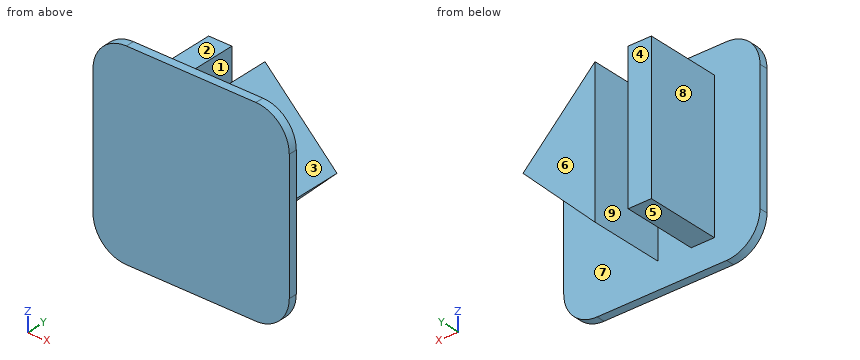
Autodesk Inventor part; units mm, degrees
ref_plane "YZ Plane" through (0, 0, 0) normal (1, 0, 0) x (0, 1, 0)
ref_plane "XZ Plane" through (0, 0, 0) normal (0, 1, 0) x (-1, 0, 0)
ref_plane "XY Plane" through (0, 0, 0) normal (0, 0, 1) x (1, 0, 0)
sketch "Szkic1" plane through (0, 0, 0) normal (0, 1, 0) x (-1, 0, 0)
  line L0 (5.1235, 4.3458) -> (-4.6765, 4.3458)
  line L1 (-4.6765, 4.3458) -> (-4.6765, -5.4542)
  line L2 (-4.6765, -5.4542) -> (5.1235, -5.4542)
  line L3 (5.1235, -5.4542) -> (5.1235, 4.3458)
  line L4 (5.1235, 4.3458) -> (-4.6765, -5.4542) construction
  line L5 (-4.6765, 4.3458) -> (5.1235, -5.4542) construction
  line L6 (0.2235, -0.5542) -> (2.6735, -0.5542)
  line L7 (3.4085, 3.8558) -> (1.9385, 3.8558)
  line L8 (1.9385, 3.8558) -> (1.9385, -4.9642)
  line L9 (1.9385, -4.9642) -> (3.4085, -4.9642)
  line L10 (3.4085, -4.9642) -> (3.4085, 3.8558)
  line L11 (3.4085, 3.8558) -> (1.9385, -4.9642) construction
  line L12 (1.9385, 3.8558) -> (3.4085, -4.9642) construction
  line L13 (0.2235, -0.5542) -> (0.0314, -0.5542)
  line L14 (0.0314, -0.5542) -> (0.0314, -4.9642)
  line L15 (0.0314, -0.5542) -> (-4.3786, -0.5542)
  line L16 (-4.3786, -0.5542) -> (0.0314, -4.9642)
  line L17 (-4.3786, -0.5542) -> (0.0314, 3.8558)
  line L18 (0.0314, -0.5542) -> (0.0314, 3.8558)
  line L19 (-5.6565, 5.3258) -> (6.1035, 5.3258)
  line L20 (6.1035, 5.3258) -> (6.1035, -6.4342)
  line L21 (6.1035, -6.4342) -> (-5.6565, -6.4342)
  line L22 (-5.6565, -6.4342) -> (-5.6565, 5.3258)
  line L23 (-5.6565, 5.3258) -> (6.1035, -6.4342) construction
  line L24 (6.1035, 5.3258) -> (-5.6565, -6.4342) construction
  point P0 (0, 0)
  dimension "d0" = 9.8
  dimension "d1" = 9.8
  dimension "d2" = 2.45
  dimension "d3" = 1.47
  dimension "d4" = 8.82
  dimension "d5" = 0.1921
  dimension "d6" = 4.41
  dimension "d7" = 4.41
  dimension "d8" = 11.76
  dimension "d9" = 11.76
extrude "Wyciągnięcie proste1" add sketch "Szkic1" along normal blind 0.5 contours L3 L2 L1 L0 | L10 L9 L8 L7 | L14 L16 L15 | L15 L17 L18 | L19 L20 L21 L22
extrude "Wyciągnięcie proste2" add sketch "Szkic1" along normal blind 5 contours L10 L9 L8 L7 | L14 L16 L15 | L15 L17 L18
fillet "Zaokrąglenie1" radius 2 4 edges at (5.6565, 0.25, 5.3258) (-6.1035, 0.25, 5.3258) (5.6565, 0.25, -6.4342) (-6.1035, 0.25, -6.4342)
offset faces "Rozmiar1" outward -0.04 faces at (-1.9385, 2, 0.9158) (-2.4285, 2, -4.9642) (-3.4085, 2, -2.0242) (-2.9185, 2, 3.8558) (-0.0314, 2, -2.0242) (1.4386, 2, 2.3858) (2.9086, 2, -2.0242)
properties part number "guzik_stop"
The model under review builds one solid part; all positions refer to its coordinate system, in mm. Face numbers are marked on the shaded views. A direction names the side the tool comes from. Coordinates: 2 decimals unless noted, no trailing zeros. Write each loop counter-clockwise with the first axis right and the second up, starting at its lowest first coordinate (ties: lowest second). Pieces come first, ordered by that corner, then holes. Notation, with made-up numbers: (25.5, -19) - (61.5, -19) arc R10 cw to (61.5, 0) - close; hole circle Ø6 at (17.5, 9). An arc over 180 degrees is marked (long way). Answer as CSV lines item,"result".
(1) We need section B-B (x = -2.5). Give the boundary of the cut face in (y, z).
Data:
outline,"(0, -6.43) - (0.5, -6.43) - (0.5, -4.92) - (5, -4.92) - (5, 3.82) - (0.5, 3.82) - (0.5, 5.33) - (0, 5.33) - close"
(2) Mouldability with a two-part tool opening along X and no side actions: class the marked faces 6, 7, 8 and 9 as pulls with the +X half, pulls with the -X half, needs draft (parallel to the pull), parting line crosses it, or undercut.
Data:
face 6,"needs draft"
face 7,"undercut"
face 8,"pulls with the -X half"
face 9,"undercut"
(3) We need section A-A (y = 2.85). Give the boundary of the cut face in (x, z), plus the area to 3 significant figures.
Data:
outline,"(-3.37, -4.92) - (-1.98, -4.92) - (-1.98, 3.82) - (-3.37, 3.82) - close; (0.01, -4.87) - (4.32, -0.55) - (0.01, 3.76) - close"
area,"30.8 mm2"
(4) We need section D-D (x = 2). Give the boundary of the cut face in (y, z), plus the area to 3 significant figures.
Data:
outline,"(0, -6.43) - (0.5, -6.43) - (0.5, -2.88) - (5, -2.88) - (5, 1.77) - (0.5, 1.77) - (0.5, 5.33) - (0, 5.33) - close"
area,"26.8 mm2"
(5) Tool access review of the marked faces 1, 2, 3, 4 and 5: name each direction out of +Z, -Z, +X, -X, +Y, -Y from which nothing blocks a thin tool from reaching the whole face with its end or side.
Data:
face 1,"+Z, -Z, +Y"
face 2,"+Z, +X, -X, +Y"
face 3,"+Z, +X, +Y"
face 4,"+Z, -Z, +X, -X, +Y"
face 5,"-Z, +X, -X, +Y"
(6) We need section C-C (z = 1.75). Give the boundary of the cut face in (x, y), plus the area to 3 significant figures.
Data:
outline,"(-6.1, 0) - (5.66, 0) - (5.66, 0.5) - (2.02, 0.5) - (2.02, 5) - (0.01, 5) - (0.01, 0.5) - (-1.98, 0.5) - (-1.98, 5) - (-3.37, 5) - (-3.37, 0.5) - (-6.1, 0.5) - close"
area,"21.2 mm2"
(7) For line 1 along Y through (x, z) = (-1.5, -1.5); line 2 along X through (y, z) = (0.7, 0.5); line 3 along X through (y, z) = (4.55, 3.5), list the stretches that pass through material, from the lowest coordinate up. Write a range as [from, to].
Data:
line 1,"y = [0, 0.5]"
line 2,"x = [-3.37, -1.98], [0.01, 3.27]"
line 3,"x = [-3.37, -1.98], [0.01, 0.27]"
(8) Clearance check with flat-ended pins moving along their axes: pin 1 Ø2 at (x, y) = (-2.5, 4) entering from +Z; pin 2 Ø2 at (y, z) = (3.5, 1.5) entering from -X; pin 3 Ø0.7 at (x, y) = (-2.5, 2) entering from -Z. State where each tip first meets the part, or that it passes through.
Data:
pin 1,"stops at z = 3.82"
pin 2,"stops at x = -3.37"
pin 3,"stops at z = -4.92"
